Build history of the part. All positions in model axes, mm. A direction names the side the tool comes from. Round coordinates to 2 decimals unless told otherwise and drop trailing zeros. Loops run counter-clockwise (first coordinate to the right, second up) from the corner with the lowest first, then second, coordinate; pieces in that order, holes last. Notation, with made-up numbers: (67, 14) - (125, 14) arc R20 cw to (125, 51) - close; hole circle Ø2 at (42, -9). An arc over 180 degrees is marked (long way). Use a Markdown table: item, result.
from build123d import *

# Parameters (mm, degrees)
SKETCH2_W           = 30
SKETCH2_H           = 30
SKETCH2_R           = 5
BOSS_EXTRUDE1_DEPTH = 20
CUT_EXTRUDE2_START  = 10
CUT_EXTRUDE2_DEPTH  = 3.7
SKETCH4_W           = 30
SKETCH4_H           = 10
SKETCH4_R           = 1.75
BOSS_EXTRUDE2_DEPTH = 5
FILLET2_R           = 3
FILLET3_R           = 1
FILLET4_R           = 2


with BuildPart() as part:
    # Sketch2 → Boss-Extrude1 (new body)
    with BuildSketch(Plane.XY):
        Rectangle(SKETCH2_W, SKETCH2_H)
        Circle(SKETCH2_R, mode=Mode.SUBTRACT)
    extrude(amount=BOSS_EXTRUDE1_DEPTH)

    # Sketch3 → Cut-Extrude2 (cut, symmetric)
    with BuildSketch(Plane.XY.offset(CUT_EXTRUDE2_START)):
        with BuildLine():
            Line((-11.2, 15), (-11.2, 0))
            ThreePointArc((-11.2, 0), (0, -11.2), (11.2, 0))
            Line((11.2, 0), (11.2, 15))
            Line((11.2, 15), (-11.2, 15))
        make_face()
    extrude(amount=CUT_EXTRUDE2_DEPTH, both=True, mode=Mode.SUBTRACT)

    # Sketch4 → Boss-Extrude2 (add)
    with BuildSketch(Plane.XZ.offset(15)):
        with Locations((0, 25)):
            Rectangle(SKETCH4_W, SKETCH4_H)
        with Locations((-12.5, 26)):
            Circle(SKETCH4_R, mode=Mode.SUBTRACT)
        with Locations((12.5, 26)):
            Circle(SKETCH4_R, mode=Mode.SUBTRACT)
    extrude(amount=-BOSS_EXTRUDE2_DEPTH)

    # Fillet2
    fillet2_edges = [part.edges().sort_by_distance(p)[0] for p in [
        (-15, -12.5, 30),
        (15, -12.5, 30),
    ]]
    fillet(fillet2_edges, radius=FILLET2_R)

    # Fillet3
    fillet3_edges = [part.edges().sort_by_distance(p)[0] for p in [
        (0, -10, 20),
    ]]
    fillet(fillet3_edges, radius=FILLET3_R)

    # Fillet4
    fillet4_edges = [part.edges().sort_by_distance(p)[0] for p in [
        (0, 15, 6.3),
        (0, 15, 13.7),
    ]]
    fillet(fillet4_edges, radius=FILLET4_R)


solid = part.part
Q1. Cut at D-D, the plane z = 11.5. List the corners of the cut face in (x, y).
Results found:
| item | result |
|---|---|
| outline | (-15, -15) - (15, -15) - (15, 15) - (11.2, 15) - (11.2, 0) arc R11.2 cw to (-11.2, 0) - (-11.2, 15) - (-15, 15) - close |
Q2. Cut at C-C, the plane y = 11.25. List the corners of the cut face in (x, z).
Results found:
| item | result |
|---|---|
| outline | (-15, 0) - (15, 0) - (15, 20) - (-15, 20) - close; hole (-11.2, 6.3) - (11.2, 6.3) - (11.2, 13.7) - (-11.2, 13.7) - close |
Q3. Drop flat-ended pins along their axis: pin 1 (4.5 mm diameter, centred on x = 12.5, z = 26, fed in from +Y); pin 2 (4 mm diameter, centred on x = 4, z = 11, fed in from +Y); pin 3 (10 mm diameter, centred on x = 4.5, z = 9.5, fed in from +Y). Give the stop position or say it passes through.
Results found:
| item | result |
|---|---|
| pin 1 | stops at y = -10 |
| pin 2 | stops at y = -9.46 |
| pin 3 | stops at y = 14.99 |
Q4. Cut at A-A, the plane z = 26. List the corners of the cut face in (x, y).
Results found:
| item | result |
|---|---|
| outline | (-15, -15) - (-14.25, -15) - (-14.25, -10) - (-15, -10) - close; (-10.75, -15) - (10.75, -15) - (10.75, -10) - (-10.75, -10) - close; (14.25, -15) - (15, -15) - (15, -10) - (14.25, -10) - close |
Q5. Probe line 1 (Y direction, x = 0, z = 2); line 2 (Z direction, x = -2.75, y = -4.75). List the from-to ranges inside material, lowest first.
Results found:
| item | result |
|---|---|
| line 1 | y = -15 to -5, 5 to 15 |
| line 2 | z = 0 to 6.3, 13.7 to 20 |
Q6. Cut at B-B, the plane x = 0. List the corners of the cut face in (y, z), plus the area to 3 significant figures.
Results found:
| item | result |
|---|---|
| outline | (-15, 0) - (-5, 0) - (-5, 6.3) - (-11.2, 6.3) - (-11.2, 13.7) - (-5, 13.7) - (-5, 20) - (-9, 20) arc R1 cw to (-10, 21) - (-10, 30) - (-15, 30) - close; (5, 0) - (15, 0) - (15, 4.3) arc R2 ccw to (13, 6.3) - (5, 6.3) - close; (5, 13.7) - (13, 13.7) arc R2 ccw to (15, 15.7) - (15, 20) - (5, 20) - close |
| area | 329 mm2 |
Q7. Pull direction Z, two halves, no side cores. Call faces 1 (the face through (14.14, -12.46, 29.1)), 2 (the face through (0, -15, 15)), 3 (the face through (12.272, -12.535, 27.735)): pulls with the +Z half, pulls with the -Z half, needs draft (parallel to the pull), parting line crosses it, or undercut.
Results found:
| item | result |
|---|---|
| face 1 | pulls with the +Z half |
| face 2 | needs draft |
| face 3 | undercut |
Q8. Which spindle directions (+Z, -Z, +X, -X, +Y, -Y) get a long thin tool onto all of the face, cutting with end or side? Do faces 4 (the face through (-14.14, -12.46, 29.1)), 5 (the face through (0, 6, 20)), 6 (the face through (-0.2, -11.2, 10.1)). Say none if no direction does.
Results found:
| item | result |
|---|---|
| face 4 | +Z, -X, +Y, -Y |
| face 5 | +Z, +X, -X, +Y |
| face 6 | +Y |
